Source: CAD feature listing. Evaluate the final solid. Frame: model axes, mm. Face numbers are marked on the shaded views. A direction names the side the tool comes from. Round coordinates to 2 decimals unless told otherwise and drop trailing zeros. Order: outer loops, then holes, each group sorted by start corner. A loop starts at its lowest first (then second) coordinate and runs counter-clockwise, first axis right, second up. Notation, with made-up numbers: (-11, -24.5) -> (-1, -24.5) arc R20 cw to (-1, 3.5) -> close; hole circle Ø8 at (-26.75, -22). An arc over 180 degrees is marked (long way). Answer as CSV lines item,"result".
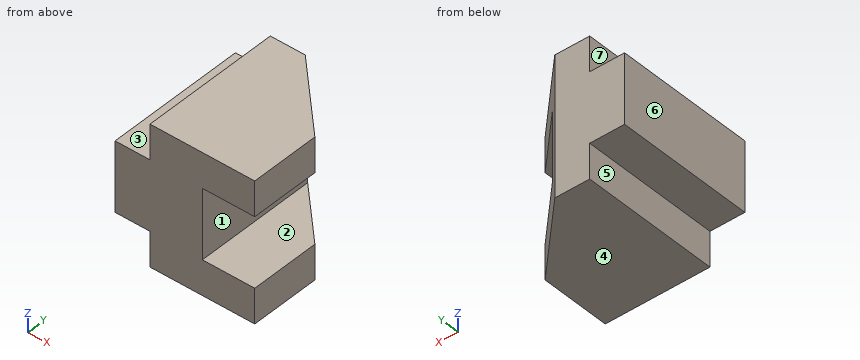
from build123d import *

# Parameters (mm, degrees)
BOSS_EXTRUDE1_DEPTH = 101.6
CUT_EXTRUDE2_DEPTH  = 102.6


with BuildPart() as part:
    # Sketch1 → Boss-Extrude1 (new body)
    with BuildSketch(Plane(origin=(0, 0, 0), x_dir=(1, 0, 0), z_dir=(0, 1, 0))):
        Polygon((0, 0), (-38.1, 0), (-38.1, 25.4), (-63.5, 25.4), (-63.5, 76.2), (-38.1, 76.2), (-38.1, 101.6), (38.1, 101.6), (38.1, 76.2), (0, 76.2), (0, 25.4), (38.1, 25.4), (38.1, 0), align=None)
    extrude(amount=BOSS_EXTRUDE1_DEPTH)

    # Sketch2 → Cut-Extrude2 (cut, through all)
    with BuildSketch(Plane.XY):
        Polygon((-12.7, 101.6), (38.1, 50.8), (38.1, 101.6), align=None)
    extrude(amount=-CUT_EXTRUDE2_DEPTH, mode=Mode.SUBTRACT)


solid = part.part
1. Section query A-A on x = 8. Return loops of the section in (y, z), and give its area (3 significant figures).
Results below:
outline,"(0, -101.6) -> (80.9, -101.6) -> (80.9, -76.2) -> (0, -76.2) -> close; (0, -25.4) -> (80.9, -25.4) -> (80.9, 0) -> (0, 0) -> close"
area,"4,110 mm2"
2. Reachability of the marked faces 5, 6 and 7 from +Z, -Z, +X, -X, +Y, -Y: full face, straight path, thin tool, end or side. Return the list, or none.
Results below:
face 5,"-Z, -X, +Y, -Y"
face 6,"+Z, -Z, -X, +Y, -Y"
face 7,"+Z, -X, +Y, -Y"
3. Section query D-D on x = -6. Return loops of the section in (y, z), and give its area (3 significant figures).
Results below:
outline,"(0, -101.6) -> (94.9, -101.6) -> (94.9, 0) -> (0, 0) -> close"
area,"9,640 mm2"
4. Line query: L1, parallel to Z at x = 26, y = 45; L2, parallel to X at y = 50.5, z = -71; L3, parallel to X at y = 48, z = -81.5. Output: solid intervals per line, ascending. Write a range as [from, to].
Results below:
L1,"[-101.6, -76.2], [-25.4, 0]"
L2,"[-63.5, 0]"
L3,"[-38.1, 38.1]"
5. Mould query, pull axis Z, two halves, no side actions, for the marked faces 1, 2, 3 and 4. Classes: released by +Z, released by -Z, zero draft, split by the parting line, or undercut.
Results below:
face 1,"undercut"
face 2,"undercut"
face 3,"released by +Z"
face 4,"released by -Z"
6. Pin query (flat end, axial travel): pin 1 (7.5 mm diameter, centred on x = -55.5, y = 60.5, fed in from -Z); pin 2 (3 mm diameter, centred on x = -45, y = 36, fed in from +Z); pin 3 (1 mm diameter, centred on x = 16, y = 31.5, fed in from +Z); pin 4 (8 mm diameter, centred on y = 13.5, z = -38.5, fed in from +X). Return the tip coordinate at first contact, or that it passes through.
Results below:
pin 1,"z = -76.2"
pin 2,"z = -25.4"
pin 3,"z = 0"
pin 4,"x = 0"
7. Section query B-B on y = 58. Return loops of the section in (x, z).
Results below:
outline,"(-63.5, -76.2) -> (-38.1, -76.2) -> (-38.1, -101.6) -> (30.9, -101.6) -> (30.9, -76.2) -> (0, -76.2) -> (0, -25.4) -> (30.9, -25.4) -> (30.9, 0) -> (-38.1, 0) -> (-38.1, -25.4) -> (-63.5, -25.4) -> close"
8. Section query C-C on z = -86. Return loops of the section in (x, y), and give its area (3 significant figures).
Results below:
outline,"(-38.1, 0) -> (38.1, 0) -> (38.1, 50.8) -> (-12.7, 101.6) -> (-38.1, 101.6) -> close"
area,"6,450 mm2"
